Could you check a few things on this model? Use its own coordinates, in mm. Face numbers are marked on the shaded views. Coordinates: 2 decimals unless noted, no trailing zeros. Loops run counter-clockwise (first coordinate to the right, second up) from the corner with the lowest first, then second, coordinate; pieces in that order, holes last. Notation, with made-up numbers: (-29, 23) - (6, 23) arc R8 ccw to (6, 38) - close; hole circle Ø9 at (21.5, 41). An arc over 180 degrees is marked (long way). One line per question, with ' | ' between items. Start each with the question number.
1. I want a section at B-B, the plane z = -56.19. Write out the boundary of the cut face in (x, y), then the cut area to 3 significant figures.
2. I want a section at D-D, the plane y = 8. Count the separate pieces of the cut face and the enclosed holes in it, then the cut area to 3 significant figures.
3. We'd pull the mould along X, two halves only. Please class the marked faces 1, 2 and 3: pulls with the +X half, pulls with the -X half, needs draft (parallel to the pull), parting line crosses it, or undercut.
4. I'm going to push a flat-ended pin straight in: P1, Ø19, axis at x = 42.25, z = -56.19, coming from the +Y side. Where does the tip first touch, or does it pass through?
5. I want a section at A-A, the plane x = 42.25. Write out the boundary of the cut face in (y, z).
6. Please list where these lines run through material, in increasing order: L1, parallel to Z at x = 42.25, y = 14.75; L2, parallel to X at y = 18.25, z = 56.19; L3, parallel to X at y = 18.25, z = -56.19. Write a range as [from, to].
7. I want a section at C-C, the plane x = 10.25. Write out the boundary of the cut face in (y, z).
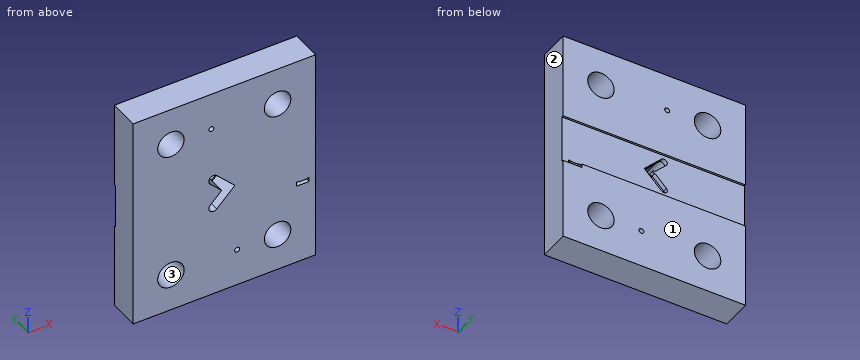
from build123d import *

# Parameters (mm, degrees)
SKETCH2_W           = 144.5
SKETCH2_H           = 172.38
BOSS_EXTRUDE1_DEPTH = 24
SKETCH3_R           = 10.5
SKETCH3_R_2         = 1.99
CUT_EXTRUDE2_DEPTH  = 25
CUT_EXTRUDE3_DEPTH  = 1.5
CUT_EXTRUDE4_DEPTH  = 19


with BuildPart() as part:
    # Sketch2 → Boss-Extrude1 (new body)
    with BuildSketch(Plane(origin=(0, 0, 0), x_dir=(1, 0, 0), z_dir=(0, 1, 0))):
        Rectangle(SKETCH2_W, SKETCH2_H)
    extrude(amount=BOSS_EXTRUDE1_DEPTH)

    # Sketch3 → Cut-Extrude2 (cut, through all)
    with BuildSketch(Plane(origin=(0, 24, 0), x_dir=(1, 0, 0), z_dir=(0, 1, 0))):
        with Locations((42.25, 56.19)):
            Circle(SKETCH3_R)
        with Locations((-42.25, 56.19)):
            Circle(SKETCH3_R)
        with Locations((-42.25, -56.19)):
            Circle(SKETCH3_R)
        with Locations((42.25, -56.19)):
            Circle(SKETCH3_R)
        with Locations((10.25, 56.19)):
            Circle(SKETCH3_R_2)
        with Locations((-10.25, -56.19)):
            Circle(SKETCH3_R_2)
        Polygon((57.25, 17.44), (59.25, 17.44), (59.25, 17.94), (65.25, 17.94), (65.25, 17.44), (67.25, 17.44), (67.25, 20.94), (57.25, 20.94), align=None)
        with BuildLine():
            Line((-10.455537495, 9.828784258), (-1.333860018, 0.707106781))
            ThreePointArc((-1.333860018, 0.707106781), (0.373246763, 0), (-1.333860018, -0.707106781))
            Line((-1.333860018, -0.707106781), (-10.455537495, -9.828784258))
            ThreePointArc((-10.455537495, -9.828784258), (-10.455537495, -13.647160877), (-6.637160877, -13.647160877))
            Line((-6.637160877, -13.647160877), (7.01, 0))
            Line((7.01, 0), (-6.637160877, 13.647160877))
            ThreePointArc((-6.637160877, 13.647160877), (-10.455537495, 13.647160877), (-10.455537495, 9.828784258))
        make_face()
    extrude(amount=-CUT_EXTRUDE2_DEPTH, mode=Mode.SUBTRACT)

    # Sketch5 → Cut-Extrude3 (cut)
    with BuildSketch(Plane(origin=(0, 24, 0), x_dir=(1, 0, 0), z_dir=(0, 1, 0))):
        Polygon((57.25, 17.94), (-72.25, 17.94), (-72.25, -17.44), (72.25, -17.44), (72.25, 20.94), (67.25, 20.94), (67.25, 17.44), (65.25, 17.44), (65.25, 17.94), (59.25, 17.94), (59.25, 17.44), (57.25, 17.44), align=None)
        with BuildLine():
            ThreePointArc((-1.333860018, -0.707106781), (0.373246763, 0), (-1.333860018, 0.707106781))
            Line((-1.333860018, 0.707106781), (-10.455537495, 9.828784258))
            ThreePointArc((-10.455537495, 9.828784258), (-10.455537495, 13.647160877), (-6.637160877, 13.647160877))
            Line((-6.637160877, 13.647160877), (7.01, 0))
            Line((7.01, 0), (-6.637160877, -13.647160877))
            ThreePointArc((-6.637160877, -13.647160877), (-10.455537495, -13.647160877), (-10.455537495, -9.828784258))
            Line((-10.455537495, -9.828784258), (-1.333860018, -0.707106781))
        make_face(mode=Mode.SUBTRACT)
    extrude(amount=-CUT_EXTRUDE3_DEPTH, mode=Mode.SUBTRACT)

    # Sketch7 → Cut-Extrude4 (cut)
    with BuildSketch(Plane.XZ):
        with BuildLine():
            Line((-2.040966799, 0), (-11.162644276, -9.121677477))
            ThreePointArc((-11.162644276, -9.121677477), (-11.162644276, -14.354267658), (-5.930054096, -14.354267658))
            Line((-5.930054096, -14.354267658), (8.424213562, 0))
            Line((8.424213562, 0), (-5.930054096, 14.354267658))
            ThreePointArc((-5.930054096, 14.354267658), (-11.162644276, 14.354267658), (-11.162644276, 9.121677477))
            Line((-11.162644276, 9.121677477), (-2.040966799, 0))
        make_face()
    extrude(amount=-CUT_EXTRUDE4_DEPTH, mode=Mode.SUBTRACT)


solid = part.part
Results are:
1) outline: (-72.25, 0) - (-52.75, 0) - (-52.75, 24) - (-72.25, 24) - close; (-31.75, 0) - (8.26, 0) - (8.26, 24) - (-31.75, 24) - close; (12.24, 0) - (31.75, 0) - (31.75, 24) - (12.24, 24) - close; (52.75, 0) - (72.25, 0) - (72.25, 24) - (52.75, 24) - close | area: 2,360 mm2
2) separate pieces: 1 | enclosed holes: 8 | area: 23,200 mm2
3) face 1: needs draft | face 2: pulls with the +X half | face 3: undercut
4) P1: passes through
5) outline: (0, -86.19) - (24, -86.19) - (24, -66.69) - (0, -66.69) - close; (0, -45.69) - (24, -45.69) - (24, -17.94) - (22.5, -17.94) - (22.5, 17.44) - (24, 17.44) - (24, 45.69) - (0, 45.69) - close; (0, 66.69) - (24, 66.69) - (24, 86.19) - (0, 86.19) - close
6) L1: z = [-86.19, -66.69], [-45.69, 45.69], [66.69, 86.19] | L2: x = [-72.25, -52.75], [-31.75, -12.24], [-8.26, 31.75], [52.75, 72.25] | L3: x = [-72.25, -52.75], [-31.75, 8.26], [12.24, 31.75], [52.75, 72.25]
7) outline: (0, -86.19) - (24, -86.19) - (24, -58.18) - (0, -58.18) - close; (0, -54.2) - (24, -54.2) - (24, -17.94) - (22.5, -17.94) - (22.5, 17.44) - (24, 17.44) - (24, 86.19) - (0, 86.19) - close
